Verification items for this drawing (mm, ordinates from the low corner). Coordinates: 2 decimals unless noted, no trailing zeros. Write each loop counter-clockwise with the first axis right and the second up, starting at its lowest first coordinate (ties: lowest second). Pieces come first, ordered by that corner, then holes. Notation, with made-up numbers: (37, -8) -> (75, -8) arc R27 cw to (75, 29) -> close; hole circle Ø11 at (-18.5, 69.5). An arc over 180 degrees is marked (long way). One line per item, written item: value. Start each with the question number.
1) Gauge pin test, flat ends, axial feed: P1, Ø12, axis at y = 31.5, z = 69.5, coming from the +X side; P2, Ø2, axis at y = 15.5, z = 131, coming from the -X side; P3, Ø2, axis at x = 40.5, y = 26, coming from the -Z side; P4, Ø1, axis at x = 84, y = 26, coming from the -Z side. Record the tip position at first contact, or that the pin passes through.
2) Scan lines: line 1 along Z through (x, y) = (75, 26.25); line 2 along Z through (x, y) = (70.5, 25); line 3 along X through (y, z) = (3.5, 53). Record each from-to range of solid material in increasing order. Write a range as [from, to].
3) Sectioned sample at C-C on y = 20. Enter the section's corners in (x, z), plus the area to 3 significant figures.
4) Sectioned sample at B-B on x = 75. Enter the section's corners in (y, z), plus the area to 3 significant figures.
5) Sectioned sample at A-A on z = 75. Enter the section's corners in (x, y).
6) Sectioned sample at D-D on y = 33. Enter the section's corners in (x, z), plus the area to 3 significant figures.
7) Draft check along X on the marked faces 1, 2 and 3. Enter one of: +X half, -X half, draft (parallel to the pull), parting line (faces both ways), or undercut.
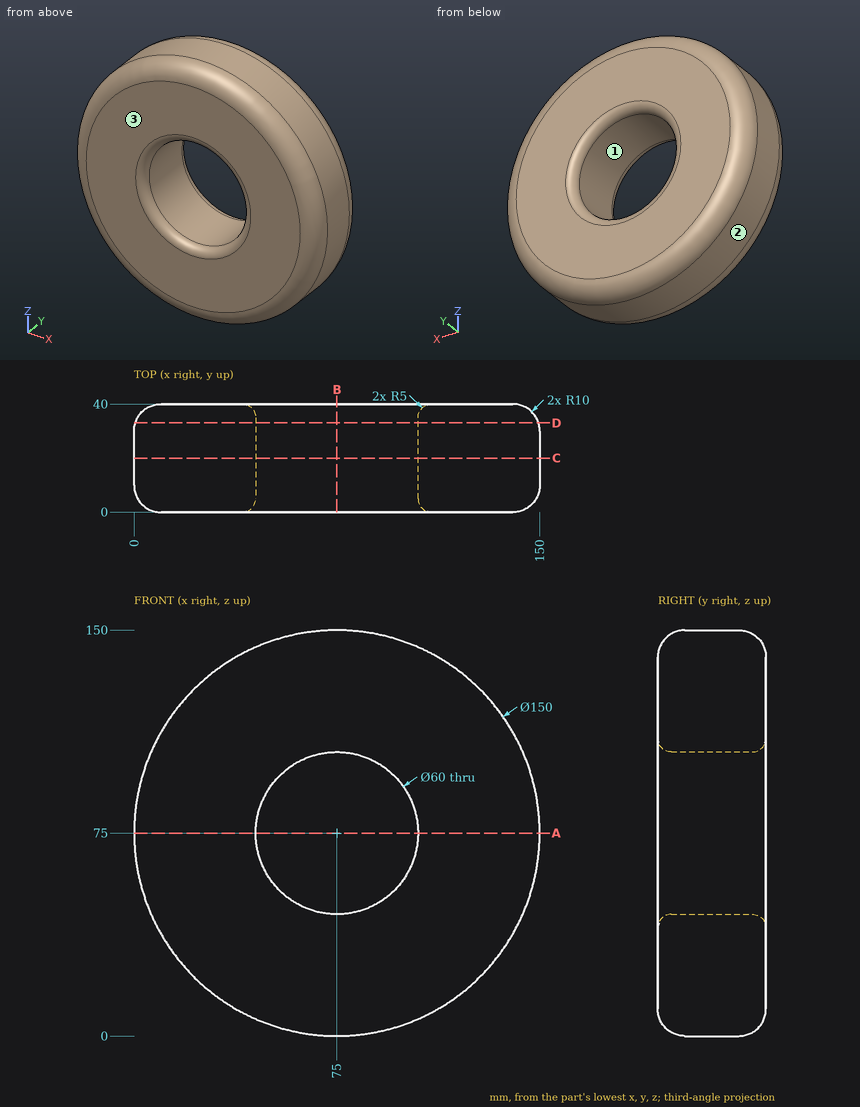
Answers:
1. P1: stops at x = 150
1. P2: stops at x = 24.01
1. P3: stops at z = 7.9
1. P4: stops at z = 0.48
2. line 1: z = [0, 45], [105, 150]
2. line 2: z = [0.14, 45.34], [104.66, 149.86]
2. line 3: x = [5.81, 54.27], [95.73, 144.19]
3. outline: circle Ø150 at (75, 75); hole circle Ø60 at (75, 75)
3. area: 14,800 mm2
4. outline: (0, 10) arc R10 ccw to (10, 0) -> (30, 0) arc R10 ccw to (40, 10) -> (40, 40) arc R5 ccw to (35, 45) -> (5, 45) arc R5 ccw to (0, 40) -> close; (0, 110) arc R5 ccw to (5, 105) -> (35, 105) arc R5 ccw to (40, 110) -> (40, 140) arc R10 ccw to (30, 150) -> (10, 150) arc R10 ccw to (0, 140) -> close
4. area: 3,490 mm2
5. outline: (0, 10) arc R10 ccw to (10, 0) -> (40, 0) arc R5 ccw to (45, 5) -> (45, 35) arc R5 ccw to (40, 40) -> (10, 40) arc R10 ccw to (0, 30) -> close; (105, 5) arc R5 ccw to (110, 0) -> (140, 0) arc R10 ccw to (150, 10) -> (150, 30) arc R10 ccw to (140, 40) -> (110, 40) arc R5 ccw to (105, 35) -> close
6. outline: circle Ø149.08 at (75, 75); hole circle Ø60 at (75, 75)
6. area: 14,600 mm2
7. face 1: undercut
7. face 2: parting line
7. face 3: draft
